Design review of the part built by this model. Coordinates are the model's own, in mm. Round coordinates to 2 decimals unless told otherwise and drop trailing zeros. Order: outer loops, then holes, each group sorted by start corner. A loop starts at its lowest first (then second) coordinate and runs counter-clockwise, first axis right, second up. Notation, with made-up numbers: M -32.5,89.25 L -18.5,89.25 A22 ccw -18.5,106.25 Z; hole C -9.75,25.5 d1. An arc over 180 degrees is marked long. Write item = value, one per line. Start each with the question number.
```python
from build123d import *

# Parameters (mm, degrees)
F0_W     = 127
F0_H     = 76.2
F0_R     = 6.35
F1_DEPTH = 50.8
F2_R     = 11.851043
F3_DEPTH = 71.628
F4_SIZE  = 12.7
F5_R     = 12.7


with BuildPart() as f1:
    # F0 (on Front) → F1 (new body)
    with BuildSketch(Plane.XZ):
        with Locations((10.547942, -5.392222)):
            Rectangle(F0_W, F0_H)
        with Locations((-37.448946, 13.657778)):
            Circle(F0_R, mode=Mode.SUBTRACT)
        with Locations((54.997942, 7.307778)):
            Circle(F0_R, mode=Mode.SUBTRACT)
    extrude(amount=F1_DEPTH)

    # F2 (on face) → F3 (cut)
    with BuildSketch(Plane.XZ.offset(50.8)):
        with Locations((20.991273, -20.324083)):
            Circle(F2_R)
    extrude(amount=-F3_DEPTH, mode=Mode.SUBTRACT)

    # F4
    f4_edges = [f1.edges().sort_by_distance(p)[0] for p in [
        (10.547942, -50.8, 32.707778),
    ]]
    chamfer(f4_edges, length=F4_SIZE)

    # F5
    f5_edges = [f1.edges().sort_by_distance(p)[0] for p in [
        (74.047942, -19.05, 32.707778),
    ]]
    fillet(f5_edges, radius=F5_R)


solid = f1.part
```
(1) For line 1 along Z through (x, y) = (55, -6); line 2 along Z through (x, y) = (-37, -22); line 3 along X through (y, z) = (-12, 12), list the stretches that pass through material, from the lowest coordinate up. Write a range as [from, to].
(2) Consider section C-C, the plane y = -5. Write out the cut boundary in (x, z), then the cut area to 3 significant figures.
(3) Consider section B-B, the plane z = -12. Write out the cut boundary in (x, y).
(4) Consider section D-D, the plane x = 2. Write out the cut boundary in (y, z).
(5) Consider section A-A, the plane x = 26. Write out the cut boundary in (y, z), then the cut area to 3 significant figures.
(6) Draft analysis for pull direction Z (two halves, no side actions). For faces 1 (the face through (9.66, -44.54, 26.27)), 2 (the face through (10, -25, -43.492)), 3 (the face through (10, 0, -5)), 4 (the face through (48.654, -25.044, 7.587)), state which applies: pulls with the +Z half, pulls with the -Z half, needs draft (parallel to the pull), parting line crosses it, or undercut.
(7) Insertion check: pin 1 (10 mm diameter, centred on x = -37.45, z = 13.66, fed in from -Y). The pin has a flat end and moves straight along its axis. Give the tip position at first contact, or say it passes through.
Completed:
q1.line_1 = [-43.49, 0.96], [13.66, 32.71]
q1.line_2 = [-43.49, 7.32], [19.99, 32.71]
q1.line_3 = [-52.95, -43.58], [-31.32, 50.72], [59.28, 74.05]
q2.outline = M -52.95,-43.49 L 74.05,-43.49 L 74.05,20.01 A12.7 ccw 61.35,32.71 L -52.95,32.71 Z; hole C -37.45,13.66 d12.7; hole C 20.99,-20.32 d23.7; hole C 55,7.31 d12.7
q2.area = 8,950 mm2
q3.outline = M -52.95,-50.8 L 12.56,-50.8 L 12.56,0 L -52.95,0 Z; M 29.43,-50.8 L 74.05,-50.8 L 74.05,0 L 29.43,0 Z
q4.outline = M -50.8,-43.49 L 0,-43.49 L 0,32.71 L -38.1,32.71 L -50.8,20.01 Z
q5.outline = M -50.8,-43.49 L 0,-43.49 L 0,-31.06 L -50.8,-31.06 Z; M -50.8,-9.58 L 0,-9.58 L 0,32.71 L -38.1,32.71 L -50.8,20.01 Z
q5.area = 2,700 mm2
q6.face_1 = pulls with the +Z half
q6.face_2 = pulls with the -Z half
q6.face_3 = needs draft
q6.face_4 = undercut
q7.pin_1 = through
